```python
from build123d import *

# Parameters (mm, degrees)
BOSS_EXTRUDE1_START = 40
MODEL_R             = 2.100000001
BOSS_EXTRUDE1_DEPTH = 406.36


with BuildPart() as part:
    # Model → Boss-Extrude1 (new body)
    with BuildSketch(Plane.XY.offset(BOSS_EXTRUDE1_START)):
        with BuildLine():
            Line((28.771485975, 48.105572105), (30.646485975, 49.980572105))
            ThreePointArc((30.646485975, 49.980572105), (30.808697649, 50.08895848), (31.000039365, 50.127018713))
            Line((31.000039365, 50.127018713), (31.592932584, 50.127018713))
            Line((31.592932584, 50.127018713), (31.592932584, 47.752018713))
            Line((31.592932584, 47.752018713), (38.292932585, 47.752018713))
            ThreePointArc((38.292932585, 47.752018713), (38.505064619, 47.664150748), (38.592932584, 47.452018714))
            Line((38.592932584, 47.452018714), (38.592932584, 45.752018713))
            Line((38.592932584, 45.752018713), (35.592932585, 45.752018713))
            Line((35.592932585, 45.752018713), (35.592932585, 44.812678885))
            Line((35.592932585, 44.812678885), (38.653592756, 41.752018713))
            Line((38.653592756, 41.752018713), (41.292932583, 41.752018713))
            Line((41.292932583, 41.752018713), (41.592932584, 41.452018713))
            Line((41.592932584, 41.452018713), (41.892932586, 41.752018714))
            Line((41.892932586, 41.752018714), (44.532272412, 41.752018714))
            Line((44.532272412, 41.752018714), (47.592932584, 44.812678886))
            Line((47.592932584, 44.812678886), (47.592932584, 45.752018714))
            Line((47.592932584, 45.752018714), (44.592932584, 45.752018714))
            Line((44.592932584, 45.752018714), (44.592932584, 47.452018715))
            ThreePointArc((44.592932584, 47.452018715), (44.68080055, 47.664150749), (44.892932584, 47.752018715))
            Line((44.892932584, 47.752018715), (61.292932583, 47.752018715))
            Line((61.292932583, 47.752018715), (61.592932582, 47.452018715))
            Line((61.592932582, 47.452018715), (61.892932583, 47.752018716))
            Line((61.892932583, 47.752018716), (71.592932583, 47.752018716))
            Line((71.592932583, 47.752018716), (71.592932583, 50.127018711))
            Line((71.592932583, 50.127018711), (72.185825802, 50.127018711))
            ThreePointArc((72.185825802, 50.127018711), (72.377167518, 50.088958477), (72.539379192, 49.980572102))
            Line((72.539379192, 49.980572102), (74.414379192, 48.105572102))
            ThreePointArc((74.414379192, 48.105572102), (74.560825801, 47.752018712), (74.414379192, 47.398465322))
            Line((74.414379192, 47.398465322), (72.539379192, 45.523465322))
            ThreePointArc((72.539379192, 45.523465322), (72.377167518, 45.415078947), (72.185825802, 45.377018714))
            Line((72.185825802, 45.377018714), (72.092932582, 45.377018714))
            ThreePointArc((72.092932582, 45.377018714), (71.739379192, 45.230572103), (71.592932583, 44.877018713))
            Line((71.592932583, 44.877018713), (71.592932583, 41.052018712))
            ThreePointArc((71.592932583, 41.052018712), (71.505064617, 40.839886678), (71.292932581, 40.752018713))
            Line((71.292932581, 40.752018713), (69.592932583, 40.752018713))
            Line((69.592932583, 40.752018713), (69.592932583, 43.752018712))
            Line((69.592932583, 43.752018712), (68.653592755, 43.752018712))
            Line((68.653592755, 43.752018712), (65.592932583, 40.691358541))
            Line((65.592932583, 40.691358541), (65.592932583, 38.052018712))
            Line((65.592932583, 38.052018712), (65.292932584, 37.752018712))
            Line((65.292932584, 37.752018712), (65.592932583, 37.452018713))
            Line((65.592932583, 37.452018713), (65.592932583, 34.812678884))
            Line((65.592932583, 34.812678884), (68.653592755, 31.752018712))
            Line((68.653592755, 31.752018712), (69.592932583, 31.752018712))
            Line((69.592932583, 31.752018712), (69.592932583, 34.752018711))
            Line((69.592932583, 34.752018711), (71.292932581, 34.752018711))
            ThreePointArc((71.292932581, 34.752018711), (71.505064617, 34.664150747), (71.592932583, 34.452018712))
            Line((71.592932583, 34.452018712), (71.592932583, 28.75201871))
            ThreePointArc((71.592932583, 28.75201871), (71.300039364, 28.044911929), (70.592932582, 27.752018711))
            Line((70.592932582, 27.752018711), (64.892932582, 27.752018711))
            ThreePointArc((64.892932582, 27.752018711), (64.680800548, 27.839886676), (64.592932583, 28.05201871))
            Line((64.592932583, 28.05201871), (64.592932583, 29.752018711))
            Line((64.592932583, 29.752018711), (67.592932582, 29.752018711))
            Line((67.592932582, 29.752018711), (67.592932582, 30.69135854))
            Line((67.592932582, 30.69135854), (64.532272411, 33.752018711))
            Line((64.532272411, 33.752018711), (61.892932584, 33.752018711))
            Line((61.892932584, 33.752018711), (61.592932582, 34.052018713))
            Line((61.592932582, 34.052018713), (61.292932582, 33.752018712))
            Line((61.292932582, 33.752018712), (58.653592755, 33.752018712))
            Line((58.653592755, 33.752018712), (55.592932583, 30.691358541))
            Line((55.592932583, 30.691358541), (55.592932583, 29.752018713))
            Line((55.592932583, 29.752018713), (58.592932583, 29.752018713))
            Line((58.592932583, 29.752018713), (58.592932583, 28.052018712))
            ThreePointArc((58.592932583, 28.052018712), (58.505064617, 27.839886678), (58.292932583, 27.752018712))
            Line((58.292932583, 27.752018712), (44.892932584, 27.752018712))
            ThreePointArc((44.892932584, 27.752018712), (44.68080055, 27.839886678), (44.592932584, 28.052018712))
            Line((44.592932584, 28.052018712), (44.592932584, 29.752018713))
            Line((44.592932584, 29.752018713), (47.592932584, 29.752018713))
            Line((47.592932584, 29.752018713), (47.592932584, 30.691358541))
            Line((47.592932584, 30.691358541), (44.532272412, 33.752018712))
            Line((44.532272412, 33.752018712), (41.892932586, 33.752018712))
            Line((41.892932586, 33.752018712), (41.592932584, 34.052018714))
            Line((41.592932584, 34.052018714), (41.292932583, 33.752018714))
            Line((41.292932583, 33.752018714), (38.653592756, 33.752018714))
            Line((38.653592756, 33.752018714), (35.592932585, 30.691358542))
            Line((35.592932585, 30.691358542), (35.592932585, 29.752018714))
            Line((35.592932585, 29.752018714), (38.592932584, 29.752018714))
            Line((38.592932584, 29.752018714), (38.592932584, 28.052018713))
            ThreePointArc((38.592932584, 28.052018713), (38.505064619, 27.839886679), (38.292932585, 27.752018714))
            Line((38.292932585, 27.752018714), (32.592932585, 27.752018714))
            ThreePointArc((32.592932585, 27.752018714), (31.885825803, 28.044911931), (31.592932584, 28.752018713))
            Line((31.592932584, 28.752018713), (31.592932584, 34.452018715))
            ThreePointArc((31.592932584, 34.452018715), (31.68080055, 34.664150748), (31.892932583, 34.752018714))
            Line((31.892932583, 34.752018714), (33.592932584, 34.752018714))
            Line((33.592932584, 34.752018714), (33.592932584, 31.752018715))
            Line((33.592932584, 31.752018715), (34.532272412, 31.752018715))
            Line((34.532272412, 31.752018715), (37.592932584, 34.812678886))
            Line((37.592932584, 34.812678886), (37.592932584, 37.452018715))
            Line((37.592932584, 37.452018715), (37.892932583, 37.752018715))
            Line((37.892932583, 37.752018715), (37.592932584, 38.052018714))
            Line((37.592932584, 38.052018714), (37.592932584, 40.691358543))
            Line((37.592932584, 40.691358543), (34.532272412, 43.752018715))
            Line((34.532272412, 43.752018715), (33.592932584, 43.752018715))
            Line((33.592932584, 43.752018715), (33.592932584, 40.752018716))
            Line((33.592932584, 40.752018716), (31.892932586, 40.752018716))
            ThreePointArc((31.892932586, 40.752018716), (31.68080055, 40.83988668), (31.592932584, 41.052018715))
            Line((31.592932584, 41.052018715), (31.592932584, 44.877018715))
            ThreePointArc((31.592932584, 44.877018715), (31.446485975, 45.230572106), (31.092932585, 45.377018716))
            Line((31.092932585, 45.377018716), (31.000039365, 45.377018716))
            ThreePointArc((31.000039365, 45.377018716), (30.808697649, 45.41507895), (30.646485975, 45.523465324))
            Line((30.646485975, 45.523465324), (28.771485975, 47.398465325))
            ThreePointArc((28.771485975, 47.398465325), (28.625039366, 47.752018715), (28.771485975, 48.105572105))
        make_face()
        with Locations((61.592932582, 37.752018715)):
            Circle(MODEL_R, mode=Mode.SUBTRACT)
        with Locations((41.592932582, 37.752018715)):
            Circle(MODEL_R, mode=Mode.SUBTRACT)
        with BuildLine():
            Line((54.092932584, 29.752018715), (49.092932584, 29.752018715))
            Line((49.092932584, 29.752018715), (49.092932584, 31.312678886))
            Line((49.092932584, 31.312678886), (45.592932583, 34.812678886))
            Line((45.592932583, 34.812678886), (45.592932583, 40.691358543))
            Line((45.592932583, 40.691358543), (49.092932584, 44.191358544))
            Line((49.092932584, 44.191358544), (49.092932584, 45.752018714))
            Line((49.092932584, 45.752018714), (67.592932582, 45.752018714))
            Line((67.592932582, 45.752018714), (67.592932582, 44.812678887))
            Line((67.592932582, 44.812678887), (64.532272411, 41.752018716))
            Line((64.532272411, 41.752018716), (61.402932584, 41.752018716))
            ThreePointArc((61.402932584, 41.752018716), (58.708855747, 40.636095552), (57.592932584, 37.942018716))
            Line((57.592932584, 37.942018716), (57.592932584, 34.812678886))
            Line((57.592932584, 34.812678886), (54.092932584, 31.312678886))
            Line((54.092932584, 31.312678886), (54.092932584, 29.752018715))
        make_face(mode=Mode.SUBTRACT)
    extrude(amount=BOSS_EXTRUDE1_DEPTH)


solid = part.part
```
Could you check a few things on this model? Use its own coordinates, in mm. A direction names the side the tool comes from. Coordinates: 2 decimals unless noted, no trailing zeros.
1) Thinking about a two-plate mould opening in Y: for faces 3 (the face through (48, 44, 446.36)), 4 (the face through (35, 47.752, 240)), 5 (the face through (58, 45.752, 240)), which applies, released by +Y, released by -Y, zero draft, split by the parting line, or undercut?
Reported:
face 3: zero draft
face 4: released by +Y
face 5: undercut
2) Will these pins go through, and if not, where does the flat tip stop? pin 1 Ø1.4 at (y, z) = (46.5, 175) entering from +X; pin 2 Ø3.5 at (x, z) = (34.5, 279.5) entering from +Y; pin 3 Ø1.5 at (y, z) = (30.5, 167) entering from -X.
Reported:
pin 1: stops at x = 74.22
pin 2: stops at y = 47.75
pin 3: stops at x = 31.59
3) Imagine slicing it at A-A (z = 285.5). State how many separate pieces and enclosed holes the cut face has, and give its area (3 significant figures).
Reported:
separate pieces: 1
enclosed holes: 3
area: 341 mm2
4) Please list where these lines run through material, in increasing order: line 1 along Y through (x, z) = (50, 166); line 2 along X through (y, z) = (40.5, 143); line 3 along X through (y, z) = (32.75, 257.5).
Reported:
line 1: y = 27.75 to 29.75, 45.75 to 47.75
line 2: x = 37.59 to 45.59, 58.58 to 65.59
line 3: x = 31.59 to 33.59, 35.53 to 37.65, 45.53 to 47.66, 55.53 to 57.65, 65.53 to 67.66, 69.59 to 71.59
5) Which directions (+Z, -Z, +X, -X, +Y, -Y) give clear straight access to the entire face, cutting with the end or side of a thin tool? Please do faces 1 (the face through (52, 27.752, 240)), 2 (the face through (67, 47.752, 240)).
Reported:
face 1: +Z, -Z, +X, -X, -Y
face 2: +Z, -Z, +Y
